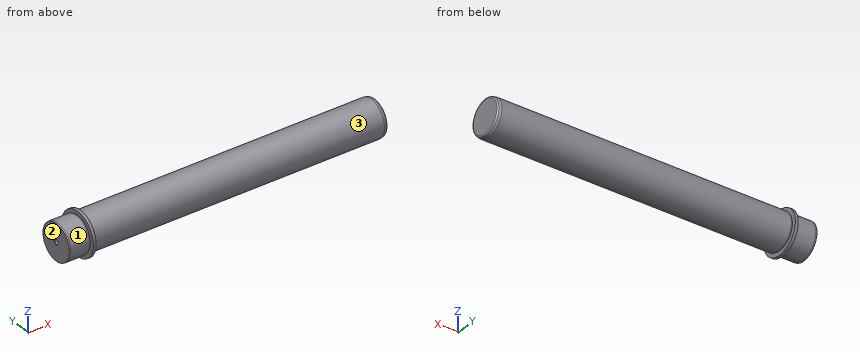
```python
from build123d import *

# Parameters (mm, degrees)
OTW_R_GWINTOWANY_M12X1_51_D           = 10.5
OTW_R_GWINTOWANY_M12X1_51_DEPTH       = 31.5
OTW_R_GWINTOWANY_M12X1_51_CSINK_D     = 12.05
OTW_R_GWINTOWANY_M12X1_51_CSINK_ANGLE = 90
OTW_R_GWINTOWANY_M12X1_51_TIP         = 3.15451825


with BuildPart() as part:
    # Sketch1 → Base-Revolve (revolve)
    with BuildSketch(Plane.XY, mode=Mode.PRIVATE) as base_revolve_sk:
        with BuildLine():
            Line((-22.233400605, 40), (18.766599395, 40))
            Line((18.766599395, 40), (18.766599395, 38.5))
            Line((18.766599395, 38.5), (21.766599395, 38.5))
            Line((21.766599395, 38.5), (21.766599395, 47.5))
            Line((21.766599395, 47.5), (28.066599395, 47.5))
            Line((28.066599395, 47.5), (28.066599395, 38.5))
            Line((28.066599395, 38.5), (31.066599395, 38.5))
            Line((31.066599395, 38.5), (31.066599395, 40))
            Line((31.066599395, 40), (666.766599395, 40))
            Line((666.766599395, 40), (672.54305653, 38.452202975))
            ThreePointArc((672.54305653, 38.452202975), (674.146659415, 37.380709784), (674.766599395, 35.554425497))
            Line((674.766599395, 35.554425497), (674.766599395, 0))
            Line((674.766599395, 0), (-25.233400605, 0))
            Line((-25.233400605, 0), (-25.233400605, 39.578377496))
            Line((-25.233400605, 39.578377496), (-22.233400605, 40))
        make_face()
    revolve(base_revolve_sk.sketch.rotate(Axis((-25.233400605, 0, 0), (1, 0, 0)), 90), axis=Axis((-25.233400605, 0, 0), (1, 0, 0)))

    # Otwór gwintowany M12x1.51
    with Locations(Plane.ZY.offset(25.233400605)):
        with Locations((0, 0)):
            CounterSinkHole(OTW_R_GWINTOWANY_M12X1_51_D / 2, OTW_R_GWINTOWANY_M12X1_51_CSINK_D / 2, depth=OTW_R_GWINTOWANY_M12X1_51_DEPTH, counter_sink_angle=OTW_R_GWINTOWANY_M12X1_51_CSINK_ANGLE)
            with Locations((0, 0, -(OTW_R_GWINTOWANY_M12X1_51_DEPTH + OTW_R_GWINTOWANY_M12X1_51_TIP / 2))):  # 118° drill point
                Cone(0, OTW_R_GWINTOWANY_M12X1_51_D / 2, OTW_R_GWINTOWANY_M12X1_51_TIP, mode=Mode.SUBTRACT)


solid = part.part
```
For this review, take the finished solid that the model builds, in its own axes (mm). Face numbers are marked on the shaded views. A direction names the side the tool comes from. Coordinates: 2 decimals unless noted, no trailing zeros. Write each loop counter-clockwise with the first axis right and the second up, starting at its lowest first coordinate (ties: lowest second). Pieces come first, ordered by that corner, then holes.
(1) Tool access review of the marked faces 1, 2 and 3: name each direction out of +Z, -Z, +X, -X, +Y, -Y from which nothing blocks a thin tool from reaching the whole face with its end or side.
(2) For pin 1 Ø6 at (x, z) = (358, 35) entering from +Y; pin 2 Ø10 at (x, y) = (471.5, -19.5) entering from -Z; pin 3 Ø4 at (x, z) = (294, -13.5) entering from +Y, all flat-tipped, find the tip position at first contact; note any pin that passes through.
(3) Add section A-A on x = 610. Give the boundary of the cut face in (y, z).
(4) Wall thickness on probe 1 along Y at (x, z) = (-3, 0); probe 2 along X at (y, z) = (28, 31); probe 3 along Z at (x, y) = (552.5, -10.5): over which ranges is each line inside the solid? List them lowest first.
Answer sheet:
1. face 1: -X
1. face 2: +Z, -Z, -X, +Y, -Y
1. face 3: +X
2. pin 1: stops at y = 24
2. pin 2: stops at z = -37.28
2. pin 3: stops at y = 38.31
3. outline: circle Ø80 at (0, 0)
4. probe 1: y = -40 to -5.25, 5.25 to 40
4. probe 2: x = 21.77 to 28.07
4. probe 3: z = -38.6 to 38.6
